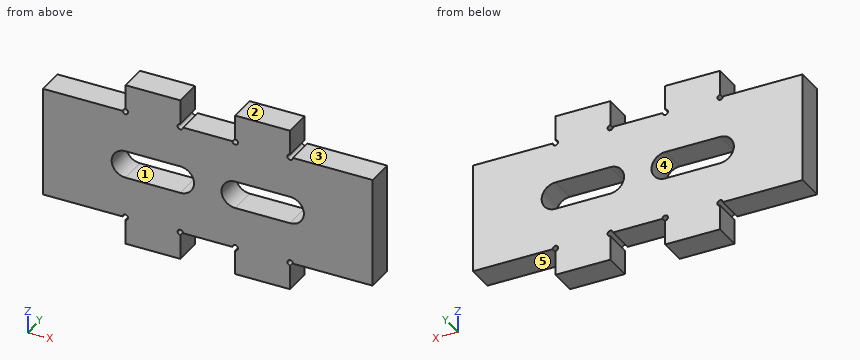
from build123d import *

# Parameters (mm, degrees)
BOSS_EXTRUDE1_DEPTH = 6.35
CUT_EXTRUDE1_REACH  = 45.068
SKETCH2_R           = 3.175
CUT_EXTRUDE2_START  = -6.35
SKETCH4_R           = 0.635
CUT_EXTRUDE2_DEPTH  = 6.35
CUT_EXTRUDE3_START  = -6.35
CUT_EXTRUDE3_DEPTH  = 6.35


with BuildPart() as part:
    # Sketch1 → Boss-Extrude1 (new body)
    with BuildSketch(Plane(origin=(0, 0, 0), x_dir=(1, 0, 0), z_dir=(0, 1, 0))):
        Polygon((-19.05, 12.7), (-19.05, 19.05), (-6.35, 19.05), (-6.35, 12.7), (6.35, 12.7), (6.35, 19.05), (19.05, 19.05), (19.05, 12.7), (38.1, 12.7), (38.1, -12.7), (19.05, -12.7), (19.05, -19.05), (6.35, -19.05), (6.35, -12.7), (-6.35, -12.7), (-6.35, -19.05), (-19.05, -19.05), (-19.05, -12.7), (-38.1, -12.7), (-38.1, 12.7), align=None)
    extrude(amount=BOSS_EXTRUDE1_DEPTH)

    # Sketch2 → Cut-Extrude1 (cut, up to next)
    with BuildSketch(Plane(origin=(0, 6.35, 0), x_dir=(1, 0, 0), z_dir=(0, 1, 0)), mode=Mode.PRIVATE) as cut_extrude1_sk1:
        with Locations(Location((-12.7, 0, 0), (0, 0, 270))):
            Circle(SKETCH2_R)
    cut_extrude1_tool1 = extrude(cut_extrude1_sk1.sketch, amount=-CUT_EXTRUDE1_REACH, mode=Mode.PRIVATE) & part.part
    # Sketch2 → Cut-Extrude1 (cut, up to next)
    with BuildSketch(Plane(origin=(0, 6.35, 0), x_dir=(1, 0, 0), z_dir=(0, 1, 0)), mode=Mode.PRIVATE) as cut_extrude1_sk2:
        with Locations(Location((12.7, 0, 0), (0, 0, 270))):
            Circle(SKETCH2_R)
    cut_extrude1_tool2 = extrude(cut_extrude1_sk2.sketch, amount=-CUT_EXTRUDE1_REACH, mode=Mode.PRIVATE) & part.part
    add(cut_extrude1_tool1.solids().sort_by_distance((-12.7, 6.35, 0))[0], mode=Mode.SUBTRACT)
    add(cut_extrude1_tool2.solids().sort_by_distance((12.7, 6.35, 0))[0], mode=Mode.SUBTRACT)

    # Sketch4 → Cut-Extrude2 (cut)
    with BuildSketch(Plane(origin=(0, 6.35, 0), x_dir=(1, 0, 0), z_dir=(0, 1, 0)).offset(CUT_EXTRUDE2_START)):
        with Locations((-19.05, 12.7)):
            Circle(SKETCH4_R)
    cut_extrude2 = extrude(amount=CUT_EXTRUDE2_DEPTH, mode=Mode.SUBTRACT)

    # Sketch-Pattern1: Cut-Extrude2 at 7 more places
    with Locations((12.7, 0, 0), (25.4, 0, 0), (38.1, 0, 0), (38.1, 0, 25.4), (25.4, 0, 25.4), (12.7, 0, 25.4), (0, 0, 25.4)):
        add(cut_extrude2, mode=Mode.SUBTRACT)

    # Sketch5 → Cut-Extrude3 (cut)
    with BuildSketch(Plane(origin=(0, 6.35, 0), x_dir=(1, 0, 0), z_dir=(0, 1, 0)).offset(CUT_EXTRUDE3_START)):
        with BuildLine():
            Line((-19.05, 3.175), (-6.35, 3.175))
            ThreePointArc((-6.35, 3.175), (-3.175, 0), (-6.35, -3.175))
            Line((-6.35, -3.175), (-19.05, -3.175))
            ThreePointArc((-19.05, -3.175), (-22.225, 0), (-19.05, 3.175))
        make_face()
        with BuildLine():
            Line((19.05, 3.175), (6.35, 3.175))
            ThreePointArc((6.35, 3.175), (3.175, 0), (6.35, -3.175))
            Line((6.35, -3.175), (19.05, -3.175))
            ThreePointArc((19.05, -3.175), (22.225, 0), (19.05, 3.175))
        make_face()
    extrude(amount=CUT_EXTRUDE3_DEPTH, mode=Mode.SUBTRACT)


solid = part.part
Build history of the part. All positions in model axes, mm. Face numbers are marked on the shaded views. A direction names the side the tool comes from. Give positions to 0.01 mm unless a question says otherwise; leave off trailing zeros. Order: outer loops, then holes, each group sorted by start corner. A loop starts at its lowest first (then second) coordinate and runs counter-clockwise, first axis right, second up. Notation, with made-up numbers: M 85.25,70.25 L 113.25,70.25 A12 ccw 113.25,85.25 Z; hole C -6.75,15.25 d5. An arc over 180 degrees is marked long. Put each result on its own line as item: value.
Item 1: Drop flat-ended pins along their axis: pin 1 Ø1 at (y, z) = (1, 13.5) entering from -X; pin 2 Ø3 at (x, y) = (-31.5, 2.5) entering from +Z; pin 3 Ø1.9 at (x, y) = (-24.5, 4.5) entering from -Z. Give the stop position or say it passes through.
Results are:
pin 1: x = -19.05
pin 2: z = 12.7
pin 3: z = -12.7
Item 2: Which spindle directions (+Z, -Z, +X, -X, +Y, -Y) get a long thin tool onto all of the face, cutting with end or side? Do the marked faces 3, 4 and 5. Say none if no direction does.
Results are:
face 3: +Z, +X, +Y, -Y
face 4: +Y, -Y
face 5: -Z, +X, +Y, -Y
Item 3: Wall check: probe 1 along X at (y, z) = (4.75, 0) (3 decimals); probe 2 along X at (y, z) = (4.5, 16); probe 3 along Z at (x, y) = (13, 1.5) (3 decimals). Give the ranges that are in metal, low to high.
Results are:
probe 1: -38.1 to -22.225, -3.175 to 3.175, 22.225 to 38.1
probe 2: -19.05 to -6.35, 6.35 to 19.05
probe 3: -19.05 to -3.175, 3.175 to 19.05
Item 4: Cut at D-D on y = 3.25. Count the separate pieces of the cut face and the enclosed holes in it, then the cut area to 3 significant figures.
Results are:
separate pieces: 1
enclosed holes: 2
area: 2,030 mm2
Item 5: Cut at B-B on z = 0. Write the cut outline in (x, y) (3 decimals), then the cut area to 3 significant figures.
Results are:
outline: M -38.1,0 L -22.225,0 L -22.225,6.35 L -38.1,6.35 Z; M -3.175,0 L 3.175,0 L 3.175,6.35 L -3.175,6.35 Z; M 22.225,0 L 38.1,0 L 38.1,6.35 L 22.225,6.35 Z
area: 242 mm2
Item 6: Pull direction X, two halves, no side cores. Call the marked faces 1 and 2: +X half, -X half, draft (parallel to the pull), parting line (faces both ways), or undercut.
Results are:
face 1: undercut
face 2: draft
Item 7: Cut at A-A on x = 12. Write the cut outline in (y, z) (3 decimals), then the cut area to 3 significant figures.
Results are:
outline: M 0,-19.05 L 6.35,-19.05 L 6.35,-3.175 L 0,-3.175 Z; M 0,3.175 L 6.35,3.175 L 6.35,19.05 L 0,19.05 Z
area: 202 mm2
